Source: CAD feature listing. Evaluate the final solid. Frame: model axes, mm. A direction names the side the tool comes from. Give positions to 0.01 mm unless a question says otherwise; leave off trailing zeros. Order: outer loops, then holes, each group sorted by start corner. A loop starts at its lowest first (then second) coordinate and runs counter-clockwise, first axis right, second up. Notation, with made-up numbers: (-36, 48.5) - (18, 48.5) arc R25 ccw to (18, 60.5) - close; hole circle Ø3 at (51.5, -19). An arc over 180 degrees is marked (long way). Answer as CSV lines item,"result".
```python
from build123d import *

# Parameters (mm, degrees)
F0_R      = 4
F1_DEPTH  = 5
F2_R      = 3
F3_DEPTH  = 2
F4_R      = 4
F4_R_2    = 3
F5_DEPTH  = 5
F6_R      = 1
F7_DEPTH  = 3
F8_R      = 2.5
F8_R_2    = 1
F9_DEPTH  = 2
F10_R     = 1
F4_R_3    = 2
F11_DEPTH = 1
F12_R     = 3.25
F13_DEPTH = 2
F14_R     = 3.5
F14_R_2   = 3.25
F15_DEPTH = 6
F16_R     = 5
F16_R_2   = 3.5
F17_DEPTH = 10
F18_R     = 3.5
F19_DEPTH = 7


with BuildPart() as f1:
    # F0 (on Front) → F1 (new body)
    with BuildSketch(Plane.XZ):
        Circle(F0_R)
    extrude(amount=F1_DEPTH)

    # F2 (on face) → F3 (join)
    with BuildSketch(Plane.XZ.offset(5)):
        Circle(F2_R)
    extrude(amount=F3_DEPTH)

    # F6 (on face) → F7 (join)
    with BuildSketch(Plane.XZ.offset(7)):
        Circle(F6_R)
    extrude(amount=F7_DEPTH)

    # F8 (on face) → F9 (join)
    with BuildSketch(Plane.XZ.offset(10)):
        Circle(F8_R)
        Circle(F8_R_2, mode=Mode.SUBTRACT)
        Circle(F8_R_2)
    extrude(amount=F9_DEPTH)

    # F10
    f10_edges = [f1.edges().sort_by_distance(p)[0] for p in [
        (-2.5, -12, 0),
    ]]
    fillet(f10_edges, radius=F10_R)



with BuildPart() as f5:
    # F4 (on face) → F5 (new body)
    with BuildSketch(Plane.XZ.offset(7)):
        Circle(F4_R)
        Circle(F4_R_2, mode=Mode.SUBTRACT)
    extrude(amount=F5_DEPTH)


with BuildPart() as f1_1:
    add(f1.part)

    add(f5.part)  # F11 merges F5
    # F4 (on face) → F11 (join)
    with BuildSketch(Plane.XZ.offset(7)):
        Circle(F4_R)
        Circle(F4_R_2, mode=Mode.SUBTRACT)
        Circle(F4_R_2)
        Circle(F4_R_3, mode=Mode.SUBTRACT)
    extrude(amount=F11_DEPTH)

    # F12 (on face) → F13 (join)
    with BuildSketch(Plane(origin=(0, 0, 0), x_dir=(-1, 0, 0), z_dir=(0, 1, 0))):
        Circle(F12_R)
    extrude(amount=F13_DEPTH)

    # F14 (on face) → F15 (join)
    with BuildSketch(Plane(origin=(0, 2, 0), x_dir=(-1, 0, 0), z_dir=(0, 1, 0))):
        Circle(F14_R)
        Circle(F14_R_2, mode=Mode.SUBTRACT)
        Circle(F14_R_2)
    extrude(amount=F15_DEPTH)

    # F16 (on face) → F17 (join)
    with BuildSketch(Plane(origin=(0, 8, 0), x_dir=(-1, 0, 0), z_dir=(0, 1, 0))):
        Circle(F16_R)
        Circle(F16_R_2, mode=Mode.SUBTRACT)
        Circle(F16_R_2)
    extrude(amount=F17_DEPTH)

    # F18 (on face) → F19 (join)
    with BuildSketch(Plane(origin=(0, 18, 0), x_dir=(-1, 0, 0), z_dir=(0, 1, 0))):
        Circle(F18_R)
    extrude(amount=F19_DEPTH)


solid = f1_1.part
```
(1) Access query for faces 1 (the flat face through (1, -5, 3)), 2 (the cylindrical face through (-0.54, -10.49, -2.44)), 3 (the cylindrical face through (1.08, 12.93, -4.88)), 4 (the cylindrical face through (-3.233, 21.451, -1.341)), 5 (the flat face through (1, -12, 3)). Directions: +Z, -Z, +X, -X, +Y, -Y. A direction counts if a zero-diameter tool reaches every point of the face in a straight line with its end or side. Return the directions, or none.
Completed:
face 1,"none"
face 2,"-Y"
face 3,"+Y, -Y"
face 4,"+Y"
face 5,"+Z, -Z, +X, -X, -Y"
(2) Contact query for flat-ended pins moving along their axis: pin 1 (1.5 mm diameter, centred on x = 1, y = 14.5, fed in from +Z); pin 2 (1.5 mm diameter, centred on y = 10, z = 4, fed in from +X); pin 3 (1.5 mm diameter, centred on x = 1, y = 5, fed in from -Z). Output: stop coordinate, or through.
Completed:
pin 1,"z = 4.99"
pin 2,"x = 3.8"
pin 3,"z = -3.49"
(3) Mould query, pull axis Z, two halves, no side actions, for faces 6 (the flat face through (1, -10, -1)), 7 (the cylindrical face through (-0.867, -9.465, -3.905)), 8 (the flat face through (-2, 0, 3)). Classes: released by +Z, released by -Z, zero draft, split by the parting line, or undercut.
Completed:
face 6,"undercut"
face 7,"split by the parting line"
face 8,"zero draft"
(4) Cut plane A-A (y = -7.5). Return loops of the section in (x, z), then the cut area to 3 significant figures.
Completed:
outline,"circle Ø8 at (0, 0); circle Ø2 at (0, 0); hole circle Ø4 at (0, 0)"
area,"40.8 mm²"
(5) Cut plane B-B (y = 16). Return loops of the section in (x, z), then the cut area to 3 significant figures.
Completed:
outline,"circle Ø10 at (0, 0)"
area,"78.5 mm²"
(6) Ray query, line 1 (Z direction, x = 0, y = -10.05); line 2 (Y direction, x = -3.25, z = 0.75); line 3 (Y direction, x = -3.5, z = 1.25). Return the intervals inside material, ascending. Write a range as from..to.
Completed:
line 1,"-4..-3, -2.5..2.5, 3..4"
line 2,"-12..-7, -5..0, 2..25"
line 3,"-12..-7, -5..0, 8..18"
